The model under review builds one solid part; all positions refer to its coordinate system, in mm. A direction names the side the tool comes from. Coordinates: 2 decimals unless noted, no trailing zeros. Loops run counter-clockwise (first coordinate to the right, second up) from the corner with the lowest first, then second, coordinate; pieces in that order, holes last. Notation, with made-up numbers: (43.25, 63) - (53.25, 63) arc R36 cw to (53.25, 101) - close; hole circle Ø3 at (-11, -9.75). An arc over 180 degrees is marked (long way). One line per item, written item: value. Start each with the question number.
1. We need section C-C, the plane x = -11. Give the boundary of the cut face in (y, z), then the cut area to 3 significant figures.
2. Mouldability with a two-part tool opening along Z and no side actions: class faces 6 (the face through (10, 10, 0)), 7 (the face through (-3.374, 8.915, 0.212)), 8 (the face through (-25, 10.8, 0)), 9 (the face through (-12.465, 10.394, -12.212)) as +Z half, -Z half, draft (parallel to the pull), parting line (faces both ways), or undercut.
3. We need section D-D, the plane z = -4.5. Give the boundary of the cut face in (x, y).
4. We need section B-B, the plane z = 0. Give the boundary of the cut face in (x, y), then the cut area to 3 significant figures.
5. We need section A-A, the plane x = 12. Give the boundary of the cut face in (y, z).
6. To check wall thickness, follow line 1 (X direction, y = 9.25, z = 0); line 2 (X direction, y = 4.5, z = 0); line 3 (X direction, y = 3, z = -1). State the ranges of each line that lie inside material, in increasing order.
7. For faces 1 (the face through (38, 6, 0)), 2 (the face through (-12.535, 10.394, 12.288)), 3 (the face through (25, 10.8, 0)), 4 (the face through (23.105, 10.394, -0.133)), 5 (the face through (-37, 13, 0)), list the 3-axis set-ups (+Z, -Z, +X, -X, +Y, -Y) from which the entire face can be reached by the end or side of a thin tool; tool diameter is ignored.
8. Insertion check: P1, Ø7.5, axis at x = -22.5, z = -2, coming from the +Y side; P2, Ø12, axis at x = 11.5, z = 0, coming from the +Y side; P3, Ø0.6, axis at x = -11.5, y = 10.5, coming from the -Z side. Each pin has a flat end and moves straight along its axis. Give the tip position at first contact, or say it passes through.
from build123d import *

# Parameters (mm, degrees)
SKETCH1_W           = 70
SKETCH1_H           = 30
BOSS_EXTRUDE1_DEPTH = 10
BOSS_EXTRUDE2_DEPTH = 0.8
CUT_EXTRUDE1_DEPTH  = 2.2
SKETCH4_R           = 2
CUT_EXTRUDE2_DEPTH  = 8
SKETCH5_W           = 3
SKETCH5_H           = 30
BOSS_EXTRUDE3_DEPTH = 13


with BuildPart() as part:
    # Sketch1 → Boss-Extrude1 (new body)
    with BuildSketch(Plane(origin=(0, 0, 0), x_dir=(1, 0, 0), z_dir=(0, 1, 0))):
        Rectangle(SKETCH1_W, SKETCH1_H)
    extrude(amount=BOSS_EXTRUDE1_DEPTH)

    # Sketch2 → Boss-Extrude2 (add)
    with BuildSketch(Plane(origin=(0, 10, 0), x_dir=(1, 0, 0), z_dir=(0, 1, 0))):
        Polygon((-15.5, -9.5), (-30.5, 9.5), (-10, 9.5), (-15, 15), (-35, 15), (-35, -15), (-15, -15), (-10, -9.5), align=None)
        Polygon((15, 15), (10, 9.5), (30.5, 9.5), (15.5, -9.5), (10, -9.5), (15, -15), (35, -15), (35, 15), align=None)
    extrude(amount=BOSS_EXTRUDE2_DEPTH)

    # Sketch3 → Cut-Extrude1 (cut)
    with BuildSketch(Plane(origin=(0, 10, 0), x_dir=(1, 0, 0), z_dir=(0, 1, 0))):
        with BuildLine():
            Line((2, 15), (2, -15))
            Line((2, -15), (-5, -15))
            ThreePointArc((-5, -15), (-3.373971656, 0), (-5, 15))
            Line((-5, 15), (2, 15))
        make_face()
    extrude(amount=-CUT_EXTRUDE1_DEPTH, mode=Mode.SUBTRACT)

    # Sketch4 → Cut-Extrude2 (cut)
    with BuildSketch(Plane(origin=(0, 10.8, 0), x_dir=(1, 0, 0), z_dir=(0, 1, 0))):
        with Locations(Location((-30, 0, 0), (0, 0, 270))):
            Circle(SKETCH4_R)
        with Locations(Location((30, 0, 0), (0, 0, 270))):
            Circle(SKETCH4_R)
    extrude(amount=-CUT_EXTRUDE2_DEPTH, mode=Mode.SUBTRACT)

    # Sketch5 → Boss-Extrude3 (add)
    with BuildSketch(Plane.XZ):
        with Locations((-36.5, 0)):
            Rectangle(SKETCH5_W, SKETCH5_H)
        with Locations((36.5, 0)):
            Rectangle(SKETCH5_W, SKETCH5_H)
    extrude(amount=-BOSS_EXTRUDE3_DEPTH)


solid = part.part
Findings below:
1. outline: (0, -15) - (10, -15) - (10, -10.6) - (10.8, -10.6) - (10.8, -9.5) - (10, -9.5) - (10, 9.5) - (10.8, 9.5) - (10.8, 10.6) - (10, 10.6) - (10, 15) - (0, 15) - close
1. area: 302 mm2
2. face 6: undercut
2. face 7: parting line
2. face 8: draft
2. face 9: -Z half
3. outline: (-38, 0) - (38, 0) - (38, 13) - (35, 13) - (35, 10.8) - (26.55, 10.8) - (26.55, 10) - (2, 10) - (2, 7.8) - (-3.52, 7.8) - (-3.52, 10) - (-26.55, 10) - (-26.55, 10.8) - (-35, 10.8) - (-35, 13) - (-38, 13) - close
4. outline: (-38, 0) - (38, 0) - (38, 13) - (35, 13) - (35, 10.8) - (32, 10.8) - (32, 2.8) - (28, 2.8) - (28, 10.8) - (23, 10.8) - (23, 10) - (2, 10) - (2, 7.8) - (-3.37, 7.8) - (-3.37, 10) - (-23, 10) - (-23, 10.8) - (-28, 10.8) - (-28, 2.8) - (-32, 2.8) - (-32, 10.8) - (-35, 10.8) - (-35, 13) - (-38, 13) - close
4. area: 721 mm2
5. outline: (0, -15) - (10, -15) - (10, -11.7) - (10.8, -11.7) - (10.8, -9.5) - (10, -9.5) - (10, 9.5) - (10.8, 9.5) - (10.8, 11.7) - (10, 11.7) - (10, 15) - (0, 15) - close
6. line 1: -38 to -32, -28 to -3.37, 2 to 28, 32 to 38
6. line 2: -38 to -32, -28 to 28, 32 to 38
6. line 3: -38 to -31.73, -28.27 to 28.27, 31.73 to 38
7. face 1: +Z, -Z, +X, +Y, -Y
7. face 2: +Z, +Y
7. face 3: +Z, -Z, +Y
7. face 4: +Y
7. face 5: +Z, -Z, +X, -X, +Y
8. P1: y = 10.8
8. P2: y = 10
8. P3: z = -11.48
